Check sheet for the modelled part. Datum: model origin and axes. Units: mm. A direction names the side the tool comes from. Give positions to 0.01 mm unless a question says otherwise; leave off trailing zeros. Loops run counter-clockwise (first coordinate to the right, second up) from the corner with the lowest first, then second, coordinate; pieces in that order, holes last. Notation, with made-up numbers: M 61.5,-11.75 L 102.5,-11.75 A22 ccw 102.5,13.25 Z; hole C 64.25,14 d11. An arc over 180 degrees is marked long. Use one line per item in the form item = value.
from build123d import *

# Parameters (mm, degrees)
SKETCH1_R           = 102.5
BOSS_EXTRUDE1_DEPTH = 20
FILLET1_R           = 10
CHAMFER1_SIZE       = 2


with BuildPart() as part:
    # Sketch1 → Boss-Extrude1 (new body)
    with BuildSketch(Plane.XY):
        Circle(SKETCH1_R)
        Polygon((23.510405521, -39.756687055), (46.18550372, 0.482264907), (22.6750982, 40.238951962), (-23.510405521, 39.756687055), (-46.18550372, -0.482264907), (-22.6750982, -40.238951962), align=None, mode=Mode.SUBTRACT)
    extrude(amount=BOSS_EXTRUDE1_DEPTH)

    # Fillet1
    fillet1_edges = [part.edges().sort_by_distance(p)[0] for p in [
        (23.510405521, -39.756687055, 10),
        (46.18550372, 0.482264907, 10),
        (22.6750982, 40.238951962, 10),
        (-23.510405521, 39.756687055, 10),
        (-46.18550372, -0.482264907, 10),
        (-22.6750982, -40.238951962, 10),
    ]]
    fillet(fillet1_edges, radius=FILLET1_R)

    # Chamfer1
    chamfer1_edges = [part.edges().sort_by_distance(p)[0] for p in [
        (-102.5, 0, 0),
        (-102.5, 0, 20),
    ]]
    chamfer(chamfer1_edges, length=CHAMFER1_SIZE)


solid = part.part
1) Section check A-A (z = 12). Record the cut outline in (x, y).
Evaluation:
outline = C 0,0 d205; hole M -43.35,4.55 A10 ccw -43.25,-5.45 L -25.61,-35.27 A10 ccw -16.9,-40.18 L 17.74,-39.82 A10 ccw 26.34,-34.73 L 43.35,-4.55 A10 ccw 43.25,5.45 L 25.61,35.27 A10 ccw 16.9,40.18 L -17.74,39.82 A10 ccw -26.34,34.73 Z
2) Section check B-B (y = 0). Record the cut outline in (x, z), then the cut area to 3 significant figures.
Evaluation:
outline = M -102.5,2 L -100.5,0 L -44.63,0 L -44.63,20 L -100.5,20 L -102.5,18 Z; M 44.63,0 L 100.5,0 L 102.5,2 L 102.5,18 L 100.5,20 L 44.63,20 Z
area = 2,310 mm^2
3) Set-up check for faces 1 (the face through (-34.73, 19.85, 9.86)), 2 (the face through (-1, -43, 0)): record each of +Z, -Z, +X, -X, +Y, -Y from which the full face is reachable in a straight line by a thin tool's end or side.
Evaluation:
face_1 = +Z, -Z
face_2 = -Z, +X, -X, +Y, -Y
4) Depth check by flat-ended pin: pin 1 Ø1 at (y, z) = (68, 2.5) entering from +X; pin 2 Ø2 at (x, z) = (-33.5, 16.5) entering from +Y; pin 3 Ø6 at (x, z) = (64.5, 6) entering from -Y. Enter the tip coordinate at first touch or a pass-through.
Evaluation:
pin_1 = 77.14
pin_2 = 97.21
pin_3 = -82
5) Section check C-C (x = 0). Record the cut outline in (y, z), then the cut area to 3 significant figures.
Evaluation:
outline = M -102.5,2 L -100.5,0 L -40,0 L -40,20 L -100.5,20 L -102.5,18 Z; M 40,0 L 100.5,0 L 102.5,2 L 102.5,18 L 100.5,20 L 40,20 Z
area = 2,490 mm^2
6) Scan lines: line 1 (Y direction, x = 13, z = 19.25); line 2 (Y direction, x = 15.5, z = 12.25); line 3 (X direction, y = -36, z = 9.5). Record each from-to range of solid material in increasing order.
Evaluation:
line_1 = -100.41 to -39.87, 40.14 to 100.41
line_2 = -101.32 to -39.84, 40.16 to 101.32
line_3 = -95.97 to -25.14, 25.49 to 95.97
7) Release check for a two-part mould opening along Y. For faces 3 (the face through (-22.22, -100.063, 9.888)), 4 (the face through (-1, -43, 20)), 5 (the face through (-21.979, -38.855, 10.14)) record: pulls with the +Y half, pulls with the -Y half, needs draft (parallel to the pull), parting line crosses it, or undercut.
Evaluation:
face_3 = parting line crosses it
face_4 = needs draft
face_5 = undercut
